Verification items for the finished model (mm, model axes). Round coordinates to 2 decimals unless told otherwise and drop trailing zeros. Write each loop counter-clockwise with the first axis right and the second up, starting at its lowest first coordinate (ties: lowest second). Pieces come first, ordered by that corner, then holes. Notation, with made-up numbers: M 6.25,9 L 12.25,9 A14 ccw 12.25,32 Z; hole C 4.5,20.5 d4. An arc over 180 degrees is marked long. Use a Markdown table: item, result. Add a question column.
Autodesk Inventor part; units mm, degrees
ref_plane "YZ Plane" through (0, 0, 0) normal (1, 0, 0) x (0, 1, 0)
ref_plane "XZ Plane" through (0, 0, 0) normal (0, 1, 0) x (-1, 0, 0)
ref_plane "XY Plane" through (0, 0, 0) normal (0, 0, 1) x (1, 0, 0)
sketch "Sketch2" plane through (0, 0, 0) normal (0, 1, 0) x (-1, 0, 0)
  circle A0 centre (0, 0) radius 60.198
  dimension "d3" = 120.396
extrude "Extrusion1" add sketch "Sketch2" along normal blind 3.175
sketch "Sketch3" plane through (0, 3.175, 0) normal (0, 1, 0) x (1, 0, 0)
  point P0 (0, 0)
  point P1 (-55.245, 0)
  point P2 (-27.6225, -47.8436)
  point P3 (27.6225, -47.8436)
  point P4 (55.245, 0)
  point P5 (27.6225, 47.8436)
  point P6 (-27.6225, 47.8436)
  dimension "d6" = 55.245
  dimension "d9" = 360
hole "Hole1" at (-55.245, 3.175, 0) at (-27.6225, 3.175, 47.8436) at (27.6225, 3.175, 47.8436) at (55.245, 3.175, 0) at (27.6225, 3.175, -47.8436) at (-27.6225, 3.175, -47.8436) direction (0, -1, 0) diameter 3 depth 25.4 tip angle 118
properties part number "Acrylic lense"
1. Depth check by flat-ended pin: pin 1 Ø1 at (x, y) = (-6, 1.5) entering from -Z; pin 2 Ø1.5 at (y, z) = (0.5, -30.5) entering from +X. Enter the tip coordinate at first touch or a pass-through.
2. Scan lines: line 1 along Z through (x, y) = (28.5, 1.3); line 2 along Z through (x, y) = (27.5, 2.6); line 3 along Z through (x, y) = (55, 0.7). Record each from-to range of solid material in increasing order. Write a range as from..to.
3. Cross-section at C-C on x = -21. Enter the section's corners in (y, z) (3 decimals), plus the area to 3 significant figures.
4. Release check for a two-part mould opening along X. For faces 1 (the cylindrical face through (13.05, 1.565, 58.767)), 2 (the flat face through (1, 0, 1)), 3 (the cylindrical face through (27.172, 1.565, 49.274)) record: +X half, -X half, draft (parallel to the pull), parting line (faces both ways), or undercut.
5. Cross-section at D-D on z = 14.5. Enter the section's corners in (x, y) (3 decimals), plus the area to 3 significant figures.
6. Cross-section at A-A on z = 0. Enter the section's corners in (x, y) (3 decimals).
7. Cross-section at B-B on y = 1. Enter the section's corners in (x, z) (1 decimal).
Answer:
| question | item | result |
|---|---|---|
| 1 | pin 1 | stops at z = -59.95 |
| 1 | pin 2 | stops at x = 52.33 |
| 2 | line 1 | z = -53.02..-49.06, -46.63..46.63, 49.06..53.02 |
| 2 | line 2 | z = -53.55..-49.34, -46.35..46.35, 49.34..53.55 |
| 2 | line 3 | z = -24.47..-1.48, 1.48..24.47 |
| 3 | outline | M 0,-56.416 L 3.175,-56.416 L 3.175,56.416 L 0,56.416 Z |
| 3 | area | 358 mm^2 |
| 4 | face 1 | parting line |
| 4 | face 2 | draft |
| 4 | face 3 | undercut |
| 5 | outline | M -58.426,0 L 58.426,0 L 58.426,3.175 L -58.426,3.175 Z |
| 5 | area | 371 mm^2 |
| 6 | outline | M -60.198,0 L -56.745,0 L -56.745,3.175 L -60.198,3.175 Z; M -53.745,0 L 53.745,0 L 53.745,3.175 L -53.745,3.175 Z; M 56.745,0 L 60.198,0 L 60.198,3.175 L 56.745,3.175 Z |
| 7 | outline | C 0,0 d120.4; hole C -55.2,0 d3; hole C -27.6,-47.8 d3; hole C -27.6,47.8 d3; hole C 27.6,-47.8 d3; hole C 27.6,47.8 d3; hole C 55.2,0 d3 |
